Autodesk Inventor part; units mm, degrees
ref_plane "YZ Plane" through (0, 0, 0) normal (1, 0, 0) x (0, 1, 0)
ref_plane "XZ Plane" through (0, 0, 0) normal (0, 1, 0) x (-1, 0, 0)
ref_plane "XY Plane" through (0, 0, 0) normal (0, 0, 1) x (1, 0, 0)
sketch "Sketch1" plane through (0, 0, 0) normal (0, 0, 1) x (1, 0, 0)
  line L0 (0, 0) -> (50.8, 0) construction
  line L1 (50.8, 0) -> (50.8, 387.35) construction
  line L2 (50.8, 387.35) -> (0, 387.35) construction
  line L3 (0, 387.35) -> (0, 0) construction
  line L4 (20.8065, 339.141) -> (-226.8638, -14.5688) construction
  line L5 (-226.8638, -14.5688) -> (-247.6703, 0) construction
  line L6 (-247.6703, 0) -> (0, 353.7099) construction
  line L7 (0, 353.7099) -> (20.8065, 339.141) construction
  line L8 (-247.6703, 0) -> (-216.6626, 0) construction
  line L9 (0, 353.7099) -> (0, 309.4263) construction
  dimension "d0" = 50.8
  dimension "d1" = 387.35
  dimension "d2" = 25.4
  dimension "d3" = 431.8
  dimension "d5" = 55
sketch "Sketch2" plane through (0, 0, 0) normal (0, 0, 1) x (1, 0, 0)
  line L0 (0, 0) -> (50.8, 0) construction
  line L1 (50.8, 0) -> (50.8, 387.35) construction
  line L2 (50.8, 387.35) -> (0, 387.35) construction
  line L3 (0, 387.35) -> (0, 0) construction
  line L4 (20.8065, 339.141) -> (-226.8638, -14.5688) construction
  line L5 (-226.8638, -14.5688) -> (-247.6703, 0) construction
  line L6 (-247.6703, 0) -> (0, 353.7099) construction
  line L7 (0, 353.7099) -> (20.8065, 339.141) construction
  line L8 (-247.6703, 0) -> (-216.6626, 0) construction
  line L9 (0, 353.7099) -> (0, 309.4263) construction
  circle A0 centre (12.7, 431.8) radius 11.176
  circle A1 centre (12.7, 431.8) radius 23.8125 construction
  circle A2 centre (12.7, 431.8) radius 39.6875 construction
  line L10 (-47.586, 285.75) -> (0, 353.7099)
  line L11 (0, 387.35) -> (0, 353.7099)
  line L12 (0, 387.35) -> (-16.2292, 404.6302)
  line L13 (52.3851, 431.368) -> (50.8, 285.75)
  line L14 (50.8, 285.75) -> (-47.586, 285.75)
  arc A3 (52.3851, 431.368) -> (-16.2292, 404.6302) centre (12.7, 431.8) ccw
  line L15 (12.7, 374.65) -> (38.1, 374.65) construction
  line L16 (10.4032, 346.4254) -> (-237.2671, -7.2844) construction
  point P0 (25.4, 0)
  point P1 (-7.8078, 320.4174)
  point P2 (-15.0922, 310.0141)
  point P3 (-22.3767, 299.6109)
  point P4 (25.4, 374.65)
  point P5 (25.4, 374.65)
  point P6 (25.4, 387.35)
  dimension "d6" = 22.352
  dimension "d7" = 47.625
  dimension "d8" = 15.875
  dimension "d10" = 12.7
  dimension "d11" = 431.8
  dimension "d12" = 101.6
  dimension "d13" = 25.4
  dimension "d14" = 12.7
  dimension "d15" = 12.7
  dimension "d16" = 12.7
  dimension "d56" = 31.75
extrude "Extrusion1" add sketch "Sketch2" along normal blind 6.35
hole "Hole1" at (0, 0, 0) at (50.8, 0, 0) at (-226.8638, -14.5688, 0) at (-247.6703, 0, 0) at (-216.6626, 0, 0) at (-7.8078, 320.4174, 0) at (-15.0922, 310.0141, 0) at (-22.3767, 299.6109, 0) at (12.7, 374.65, 0) at (25.4, 374.65, 0) at (38.1, 374.65, 0) direction (0, 0, 1) diameter 3.9624 end through all
fillet "Fillet1" radius 6.604 3 edges at (0, 353.7099, 3.175) (-47.586, 285.75, 3.175) (50.8, 285.75, 3.175)
sketch "Sketch3" plane through (0, 0, 0) normal (0, 0, -1) x (-1, 0, 0)
  arc A0 (-50.8711, 292.2821) -> (-44.2675, 285.75) centre (-44.2675, 292.354) ccw construction
  line L0 (34.8998, 285.75) -> (-44.2675, 285.75) construction
  arc A1 (34.8998, 285.75) -> (40.3095, 296.1419) centre (34.8998, 292.354) ccw construction
  line L1 (1.1943, 352.0042) -> (40.3095, 296.1419) construction
  arc A2 (0, 355.7921) -> (1.1943, 352.0042) centre (6.604, 355.7921) ccw construction
  line L2 (0, 387.35) -> (0, 355.7921) construction
  line L3 (16.2292, 404.6302) -> (0, 387.35) construction
  arc A3 (16.2292, 404.6302) -> (-52.3851, 431.368) centre (-12.7, 431.8) ccw construction
  line L4 (-50.8711, 292.2821) -> (-52.3851, 431.368) construction
  circle A4 centre (-25.4, 374.65) radius 1.9812 construction
  circle A5 centre (22.3767, 299.6109) radius 1.9812 construction
  circle A6 centre (7.8078, 320.4174) radius 1.9812 construction
  circle A7 centre (15.0922, 310.0141) radius 1.9812 construction
  circle A8 centre (-12.7, 374.65) radius 1.9812 construction
  circle A9 centre (-38.1, 374.65) radius 1.9812 construction
  circle A10 centre (-12.7, 431.8) radius 11.176 construction
  circle A11 centre (-12.7, 431.8) radius 23.8125
  circle A12 centre (-12.7, 431.8) radius 11.176 construction
  circle A13 centre (-12.7, 431.8) radius 31.75 construction
  point P0 (0, 0)
  point P1 (-12.7, 463.55)
  point P2 (-44.45, 431.8)
  point P3 (-12.7, 400.05)
  point P4 (19.05, 431.8)
  dimension "d29" = 63.5
  dimension "d28" = 47.625
  dimension "d32" = 360
extrude "Extrusion2" cut sketch "Sketch3" against normal blind 3.175
hole "Hole2" at (12.7, 463.55, 0) at (44.45, 431.8, 0) at (12.7, 400.05, 0) at (-19.05, 431.8, 0) direction (0, 0, 1) diameter 3.9624 end through all
sketch "Sketch4" plane through (0, 0, 6.35) normal (0, 0, 1) x (1, 0, 0)
  line L0 (-1.1943, 352.0042) -> (-40.3095, 296.1419)
  line L1 (-12.0155, 336.55) -> (51.353, 336.55)
  line L2 (50.8711, 292.2821) -> (52.3851, 431.368)
  line L3 (-34.8998, 285.75) -> (44.2675, 285.75)
  arc A0 (-40.3095, 296.1419) -> (-34.8998, 285.75) centre (-34.8998, 292.354) ccw
  arc A1 (44.2675, 285.75) -> (50.8711, 292.2821) centre (44.2675, 292.354) ccw
  point P0 (0, 0)
  dimension "d43" = 50.8
extrude "Extrusion3" cut sketch "Sketch4" against normal through all keep common part
fillet "Fillet2" radius 3.175 2 edges at (-12.0155, 336.55, 3.175) (51.353, 336.55, 3.175)
sketch "Sketch5" plane through (0, 0, 6.35) normal (0, 0, 1) x (1, 0, 0)
  line L0 (50.8, 387.35) -> (0, 387.35) construction
  line L1 (25.4, 323.85) -> (25.4, 298.45) construction
  line L2 (-34.8998, 285.75) -> (44.2675, 285.75) construction
  point P0 (0, 0)
  point P1 (25.4, 387.35)
  dimension "d47" = 25.4
  dimension "d48" = 12.7
hole "Hole3" at (25.4, 323.85, 6.35) at (25.4, 298.45, 6.35) direction (0, 0, -1) diameter 3.9624 end through all
properties part number "CL7-011" material "Aluminum 6061"
Design review of the part built by this model. Coordinates are the model's own, in mm. Give positions to 0.01 mm unless a question says otherwise; leave off trailing zeros. Loops run counter-clockwise (first coordinate to the right, second up) from the corner with the lowest first, then second, coordinate; pieces in that order, holes last. Notation, with made-up numbers: (28.25, 56) -> (77.25, 56) arc R33 cw to (77.25, 95) -> close; hole circle Ø4 at (88.5, 45). An arc over 180 degrees is marked (long way). One line per item, written item: value.
Q1. We need section D-D on y = 299. Give the boundary of the cut face in (x, z).
Numbers:
outline: (-38.31, 0) -> (-24.26, 0) -> (-24.26, 6.35) -> (-38.31, 6.35) -> close; (-20.49, 0) -> (23.5, 0) -> (23.5, 6.35) -> (-20.49, 6.35) -> close; (27.3, 0) -> (50.94, 0) -> (50.94, 6.35) -> (27.3, 6.35) -> close
Q2. Draft analysis for pull direction X (two halves, no side actions). For faces 1 (the cylindrical face through (-22.46, 297.63, 3.22)), 2 (the cylindrical face through (48.86, 287.61, 3.22)), 3 (the flat face through (-26.828, 315.396, 3.131)), state which applies: pulls with the +X half, pulls with the -X half, needs draft (parallel to the pull), parting line crosses it, or undercut.
Numbers:
face 1: undercut
face 2: pulls with the +X half
face 3: pulls with the -X half
Q3. We need section C-C on z = 4.5. Give the number of separate pieces and of enclosed holes in the cut face, and give its area (3 significant figures).
Numbers:
separate pieces: 1
enclosed holes: 5
area: 4,000 mm^2
Q4. For L1, parallel to Y at x = 25.4, z = 1.5; L2, parallel to X at y = 298.45, z = 2.25; L3, parallel to X at y = 309, z = 1.75, list the stretches that pass through material, from the lowest coordinate up.
Numbers:
L1: y = 285.75 to 296.47, 300.43 to 321.87, 325.83 to 336.55
L2: x = -38.69 to -23.98, -20.77 to 23.42, 27.38 to 50.94
L3: x = -31.31 to -16.79, -13.39 to 51.05
Q5. For pin 1 Ø2 at (y, z) = (301, 3.5) entering from -X, flat-tipped, find the tip position at first contact; note if it passes through.
Numbers:
pin 1: stops at x = -37.61
Q6. We need section A-A on x = 25.4. Give the boundary of the cut face in (y, z).
Numbers:
outline: (285.75, 0) -> (296.47, 0) -> (296.47, 6.35) -> (285.75, 6.35) -> close; (300.43, 0) -> (321.87, 0) -> (321.87, 6.35) -> (300.43, 6.35) -> close; (325.83, 0) -> (336.55, 0) -> (336.55, 6.35) -> (325.83, 6.35) -> close
Q7. We need section B-B on y = 323.85. Give the boundary of the cut face in (x, z).
Numbers:
outline: (-20.91, 0) -> (23.42, 0) -> (23.42, 6.35) -> (-20.91, 6.35) -> close; (27.38, 0) -> (51.21, 0) -> (51.21, 6.35) -> (27.38, 6.35) -> close
